Verification items for the finished model (mm, model axes). Face numbers are marked on the shaded views. A direction names the side the tool comes from. Coordinates: 2 decimals unless noted, no trailing zeros. Write each loop counter-clockwise with the first axis right and the second up, starting at its lowest first coordinate (ties: lowest second). Pieces come first, ordered by that corner, then holes. Notation, with made-up numbers: (51.5, 32) -> (79.5, 32) arc R31 ccw to (79.5, 63) -> close; hole circle Ø6 at (-20.5, -13). An arc over 180 degrees is marked (long way). Write each question's results on one line, items separated by ' | '. Start each with the question number.
from build123d import *

# Parameters (mm, degrees)
F1_DEPTH = 35
F2_W     = 163.409721
F2_H     = 173.085335
F3_DEPTH = 20
F4_R     = 17.5
F5_DEPTH = 100


with BuildPart() as f1:
    # F0 (on Right) → F1 (new body, symmetric)
    with BuildSketch(Plane.YZ):
        with BuildLine():
            Line((0, 37.721872), (0, 0))
            Line((0, 0), (0, -20))
            Line((0, -20), (84.224192, 1.374048))
            ThreePointArc((84.224192, 1.374048), (112.5, 37.721872), (84.224192, 74.069695))
            Line((84.224192, 74.069695), (0, 95.443744))
            Line((0, 95.443744), (0, 75.443744))
            Line((0, 75.443744), (0, 37.721872))
        make_face()
    extrude(amount=F1_DEPTH, both=True)

    # F2 (on Right) → F3 (cut, symmetric)
    with BuildSketch(Plane.YZ):
        with Locations((101.70486, 41.636539)):
            Rectangle(F2_W, F2_H)
    extrude(amount=F3_DEPTH, both=True, mode=Mode.SUBTRACT)

    # F4 (on face) → F5 (cut)
    with BuildSketch(Plane.YZ.offset(35)):
        with Locations((75, 37.721872)):
            Circle(F4_R)
    extrude(amount=-F5_DEPTH, mode=Mode.SUBTRACT)


solid = f1.part
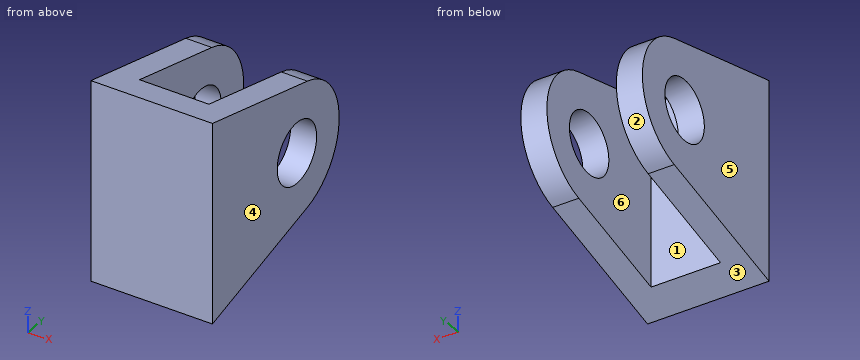
1. Mould release check, pull along X, two halves, no side actions. Record for the marked faces 3, 4, 5 and 6: +X half, -X half, draft (parallel to the pull), parting line (faces both ways), or undercut.
2. Material ranges on probe 1 along X at (y, z) = (30.5, 77.5); probe 2 along Y at (x, z) = (-5, 49); probe 3 along Y at (x, z) = (-32, 36), recorded low to high. Write a range as from..to.
3. Sectioned sample at D-D on z = 17. Record the cut outline in (x, y), plus the area to 3 significant figures.
4. Sectioned sample at B-B on y = 26. Record the cut outline in (x, z).
5. Sectioned sample at C-C on y = 75. Record the cut outline in (x, z), plus the area to 3 significant figures.
6. Sectioned sample at A-A on z = 33.5. Record the cut outline in (x, y).
7. Tool access check on the marked faces 1 and 2. Record the directions out of +Z, -Z, +X, -X, +Y, -Y that give a thin tool (end or side, any length) a straight path to the whole face; none if there is none.
8. Depth check by flat-ended pin: pin 1 Ø3 at (x, y) = (21.5, 58) entering from +Z; pin 2 Ø8 at (x, z) = (2.5, -2.5) entering from +Y; pin 3 Ø4 at (x, z) = (-20.5, 66) entering from +Y. Enter the tip coordinate at first touch or a pass-through.
Computed values:
1) face 3: draft | face 4: +X half | face 5: -X half | face 6: undercut
2) probe 1: x = -35..-20, 20..35 | probe 2: y = 0..20 | probe 3: y = 0..57.58, 92.42..112.46
3) outline: (-35, 0) -> (35, 0) -> (35, 106.25) -> (20, 106.25) -> (20, 20) -> (-20, 20) -> (-20, 106.25) -> (-35, 106.25) -> close | area: 3,990 mm^2
4) outline: (-35, -13.4) -> (-20, -13.4) -> (-20, 88.85) -> (-35, 88.85) -> close; (20, -13.4) -> (35, -13.4) -> (35, 88.85) -> (20, 88.85) -> close
5) outline: (-35, -0.97) -> (-20, -0.97) -> (-20, 20.22) -> (-35, 20.22) -> close; (-35, 55.22) -> (-20, 55.22) -> (-20, 76.41) -> (-35, 76.41) -> close; (20, -0.97) -> (35, -0.97) -> (35, 20.22) -> (20, 20.22) -> close; (20, 55.22) -> (35, 55.22) -> (35, 76.41) -> (20, 76.41) -> close | area: 1,270 mm^2
6) outline: (-35, 0) -> (35, 0) -> (35, 58.02) -> (20, 58.02) -> (20, 20) -> (-20, 20) -> (-20, 58.02) -> (-35, 58.02) -> close; (-35, 91.98) -> (-20, 91.98) -> (-20, 112.26) -> (-35, 112.26) -> close; (20, 91.98) -> (35, 91.98) -> (35, 112.26) -> (20, 112.26) -> close
7) face 1: +Z, -Z, +Y | face 2: +X, -X, +Y
8) pin 1: stops at z = 81.11 | pin 2: stops at y = 20 | pin 3: stops at y = 101.75
